Can you work these out from the drawing? Everything is in mm from the part's minimum corner. A direction names the side the tool comes from. Round coordinates to 2 decimals unless told otherwise and drop trailing zeros. Write each loop counter-clockwise with the first axis right and the second up, starting at its lowest first coordinate (ties: lowest second). Pieces come first, ordered by that corner, then holes. Notation, with made-up numbers: (-12.75, -2.75) -> (32.25, -2.75) arc R23 ccw to (32.25, 27.25) -> close; hole circle Ø10 at (-22.5, 11). An arc over 180 degrees is marked (long way). Write item = value, one per line. Start each with the question number.
1) Imagine slicing it at C-C, the plane z = 7.5. Please give me the cut outline in (x, y), then the cut area to 3 significant figures.
2) I'm going to push flat-ended pins straight in: pin 1 (3 mm diameter, centred on x = 15, z = 10.5, fed in from +Y); pin 2 (2 mm diameter, centred on x = 13, z = 13.5, fed in from +Y); pin 3 (3 mm diameter, centred on y = 2.5, z = 4.5, fed in from -X). Where does each tip first touch, or does it pass through?
3) For the marked faces 1 and 2, which set-ups out of +Z, -Z, +X, -X, +Y, -Y let a thin tool reach every point of the face, with its end or its side?
4) Imagine slicing it at B-B, the plane z = 32.5. Please give me the cut outline in (x, y), then the cut area to 3 significant figures.
5) Imagine slicing it at A-A, the plane x = 10. Please give me the cut outline in (y, z), then the cut area to 3 significant figures.
6) If I drill on line 1 (Z direction, x = 1, y = 10.75); line 2 (Z direction, x = 18, y = 4.5); line 3 (Y direction, x = 17.5, z = 4), over which ranges is the centre line in solid material (lowest first)?
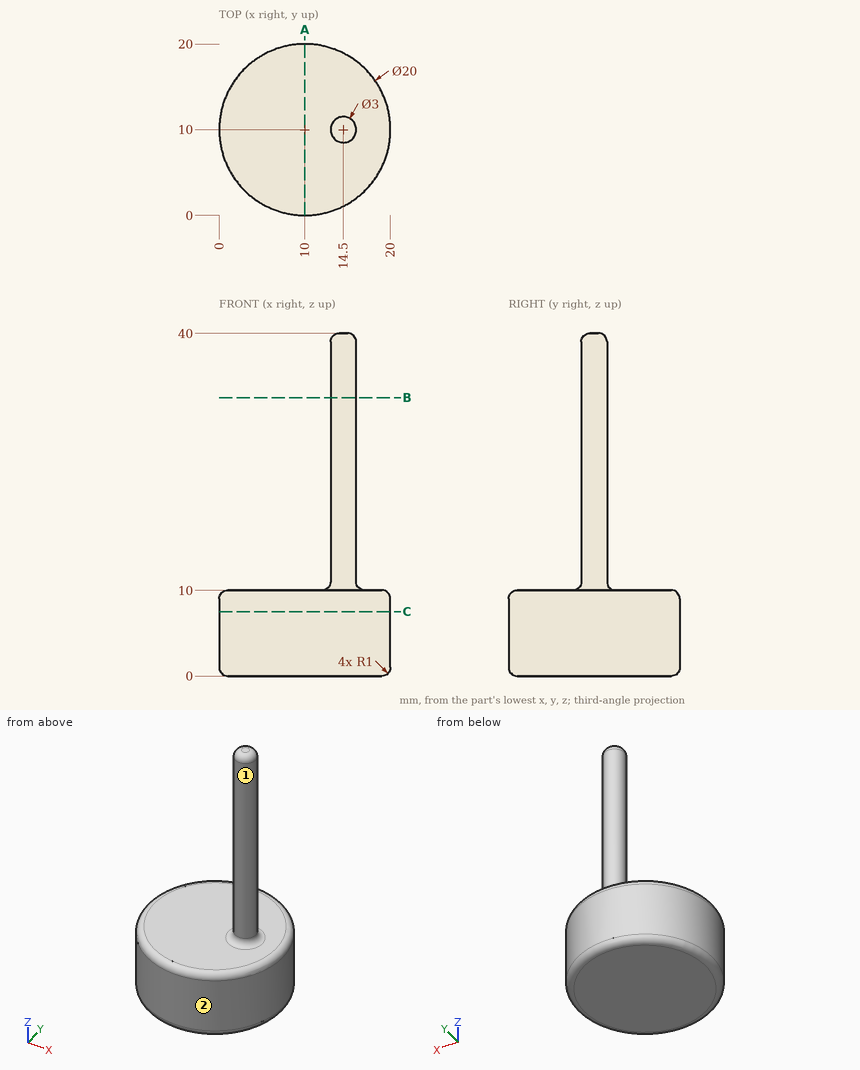
Reported:
q1.outline = circle Ø20 at (10, 10)
q1.area = 314 mm²
q2.pin_1 = 19.08
q2.pin_2 = 11.41
q2.pin_3 = 2
q3.face_1 = +Z
q3.face_2 = +Z, -Z
q4.outline = circle Ø3 at (14.5, 10)
q4.area = 7.07 mm²
q5.outline = (0, 1) arc R1 ccw to (1, 0) -> (19, 0) arc R1 ccw to (20, 1) -> (20, 9) arc R1 ccw to (19, 10) -> (1, 10) arc R1 ccw to (0, 9) -> close
q5.area = 199 mm²
q6.line_1 = 0 to 10
q6.line_2 = 0.29 to 9.71
q6.line_3 = 3.39 to 16.61
